Source: three-view drawing plus pictorial views. Frame: mm from the lowest corner of the part. A direction names the side the tool comes from. Coordinates: 2 decimals unless noted, no trailing zeros. Order: outer loops, then holes, each group sorted by start corner. A loop starts at its lowest first (then second) coordinate and runs counter-clockwise, first axis right, second up. Notation, with made-up numbers: (-31.75, 23.25) -> (-20.75, 23.25) arc R34 ccw to (-20.75, 57.25) -> close; hole circle Ø1 at (-13, 25.25). An arc over 180 degrees is marked (long way). Use one line per item in the form item = value. Start each with the question number.
1) Pin query (flat end, axial travel): pin 1 (4 mm diameter, centred on x = 20, z = 5, fed in from +Y); pin 2 (1 mm diameter, centred on x = 14.5, y = 4.5, fed in from -Z); pin 3 (2 mm diameter, centred on x = 22.5, y = 11, fed in from -Z). Return the tip coordinate at first contact, or that it passes through.
2) Section query B-B on x = 13.25. Output: boundary loops of the cut face in (y, z) (3 decimals), then the cut area to 3 significant figures.
3) Draft query along Z for the marked faces 1, 2, 3 and 4. Return one class per face: pulls with the +Z half, pulls with the -Z half, needs draft (parallel to the pull), parting line crosses it, or undercut.
4) Section query D-D on z = 42. Output: boundary loops of the cut face in (x, y).
5) Section query C-C on z = 51.5. Output: boundary loops of the cut face in (x, y).
6) Ray query, line 1 along Z through (x, y) = (19, 3.25) (1 decimal); line 2 along X through (y, z) = (13, 6.5); line 3 along X through (y, z) = (10.75, 50). Return the intervals inside material, ascending.
7) Access query for the marked faces 5 and 6. Directions: +Z, -Z, +X, -X, +Y, -Y. A direction counts if a zero-diameter tool reaches every point of the face in a straight line with its end or side. Return the directions, or none.
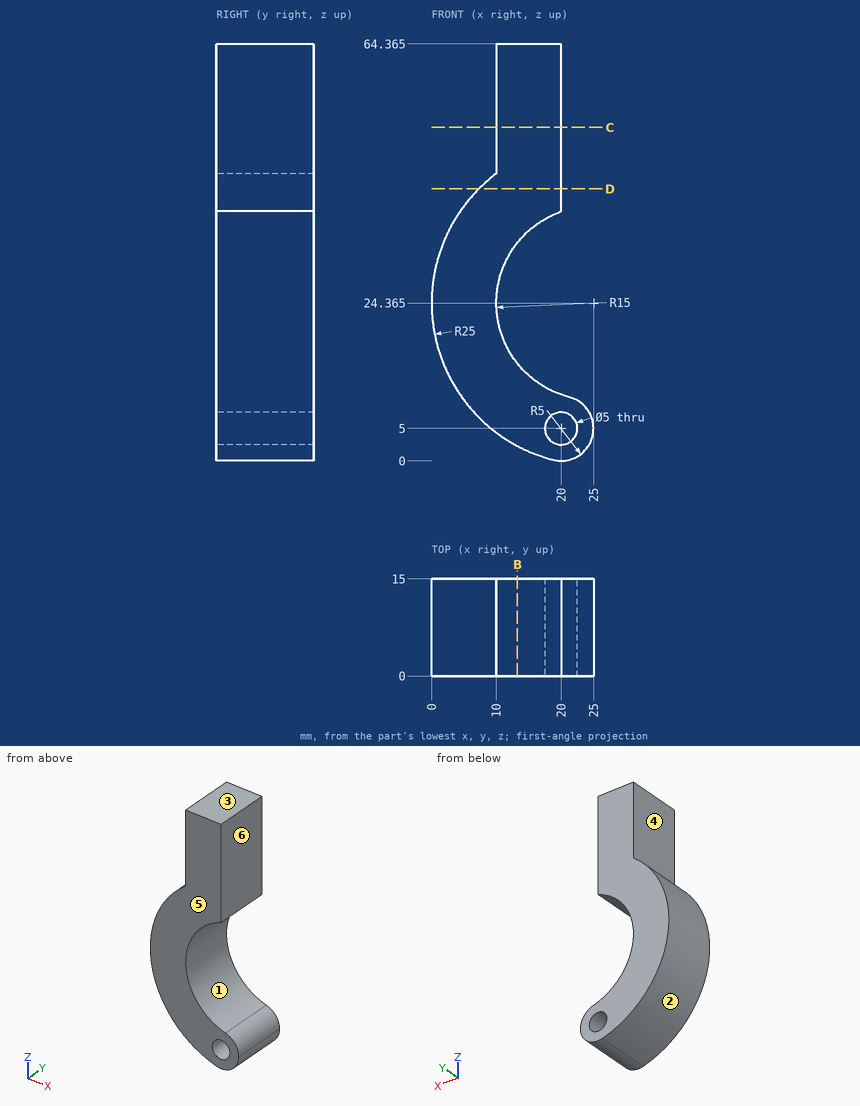
Answers below:
q1.pin_1 = through
q1.pin_2 = 1.45
q1.pin_3 = 0.23
q2.outline = (0, 2.298) -> (15, 2.298) -> (15, 15.041) -> (0, 15.041) -> close; (0, 33.689) -> (15, 33.689) -> (15, 64.365) -> (0, 64.365) -> close
q2.area = 651 mm^2
q3.face_1 = undercut
q3.face_2 = parting line crosses it
q3.face_3 = pulls with the +Z half
q3.face_4 = needs draft
q4.outline = (7.28, 0) -> (20, 0) -> (20, 15) -> (7.28, 15) -> close
q5.outline = (10, 0) -> (20, 0) -> (20, 15) -> (10, 15) -> close
q6.line_1 = 0.1 to 2.7, 7.3 to 10.6, 38.1 to 64.4
q6.line_2 = 7.51 to 18, 22 to 24.77
q6.line_3 = 10 to 20
q7.face_5 = +Z, -Z, +X, -X, -Y
q7.face_6 = +Z, +X, +Y, -Y
